```python
from build123d import *

# Parameters (mm, degrees)
F0_R     = 12.5
F1_DEPTH = 5
F2_R     = 10


with BuildPart() as f1:
    # F0 (on Front) → F1 (new body)
    with BuildSketch(Plane.XZ):
        Polygon((25, 43.30127), (0, 0), (50, 0), align=None)
        with Locations((25, 15.30127)):
            Circle(F0_R, mode=Mode.SUBTRACT)
    extrude(amount=F1_DEPTH)

    # F2
    f2_edges = [f1.edges().sort_by_distance(p)[0] for p in [
        (25, -2.5, 43.30127),
        (0, -2.5, 0),
        (50, -2.5, 0),
    ]]
    fillet(f2_edges, radius=F2_R)


solid = f1.part
```
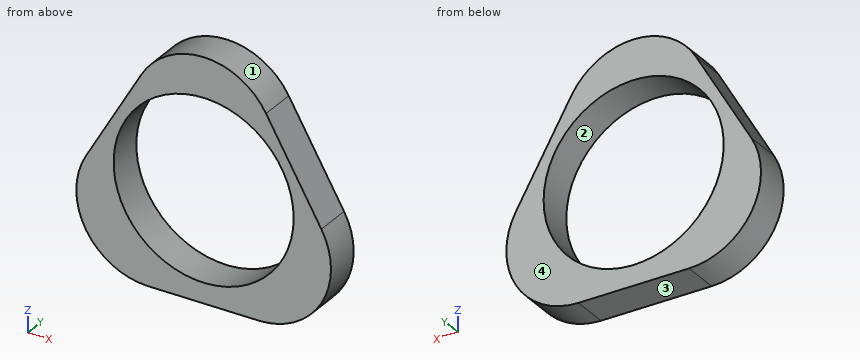
Part model, mm, in its own coordinate system. Face numbers are marked on the shaded views. Round coordinates to 2 decimals unless told otherwise and drop trailing zeros. Write each loop counter-clockwise with the first axis right and the second up, starting at its lowest first coordinate (ties: lowest second). Pieces come first, ordered by that corner, then holes. Notation, with made-up numbers: (-33.75, 11) -> (-27.75, 11) arc R13 ccw to (-27.75, 24) -> close; hole circle Ø7 at (-28.5, -21). An arc over 180 degrees is marked (long way). Return JSON: item names as keys, results as strings. Group by question number.
Q1. Mould opens along Z. For the marked faces 1, 2, 3 and 4 say: pulls with the +Z half, pulls with the -Z half, needs draft (parallel to the pull), parting line crosses it, or undercut.
Q2. Saw through at A-A on x = 25. Write the cut outline in (y, z).
Q3. Pin check, flat tips, straight feed: pin 1 (1 mm diameter, centred on x = 33.5, y = -2, fed in from -Z); pin 2 (2 mm diameter, centred on x = 11, y = -3, fed in from +Z); pin 3 (8 mm diameter, centred on x = 22, z = 22.5, fed in from -Y) (3 decimals); pin 4 (2 mm diameter, centred on y = -2, z = 14, fed in from +X). Stop position of each tip, or through.
Q4. Saw through at D-D on x = 40. Write the cut outline in (y, z), plus the area to 3 significant figures.
Q5. Probe L1, parallel to Z at x = 25, y = -3.65; L2, parallel to Z at x = 28, y = -1.7; L3, parallel to X at y = -2.65, z = 24. List the from-to ranges inside material, lowest first. Write a range as [from, to].
Q6. Saw through at B-B on z = 22. Write the cut outline in (x, y).
Q7. Saw through at C-C on y = -2.85. Write the cut outline in (x, z), plus the area to 3 significant figures.
Answer:
{
 "1": {"face 1": "pulls with the +Z half", "face 2": "undercut", "face 3": "pulls with the -Z half", "face 4": "needs draft"},
 "2": {"outline": "(-5, 0) -> (0, 0) -> (0, 2.8) -> (-5, 2.8) -> close; (-5, 27.8) -> (0, 27.8) -> (0, 33.3) -> (-5, 33.3) -> close"},
 "3": {"pin 1": "z = 0.01", "pin 2": "z = 20.78", "pin 3": "through", "pin 4": "x = 42.22"},
 "4": {"outline": "(-5, 3.19) -> (0, 3.19) -> (0, 17.32) -> (-5, 17.32) -> close", "area": "70.7 mm2"},
 "5": {"L1": "[0, 2.8], [27.8, 33.3]", "L2": "[0, 3.17], [27.44, 32.84]", "L3": "[13.86, 16.02], [33.98, 36.14]"},
 "6": {"outline": "(12.7, -5) -> (14.45, -5) -> (14.45, 0) -> (12.7, 0) -> close; (35.55, -5) -> (37.3, -5) -> (37.3, 0) -> (35.55, 0) -> close"},
 "7": {"outline": "(8.66, 15) arc R10 ccw to (17.32, 0) -> (32.68, 0) arc R10 ccw to (41.34, 15) -> (33.66, 28.3) arc R10 ccw to (16.34, 28.3) -> close; hole circle Ø25 at (25, 15.3)", "area": "386 mm2"}
}
